from build123d import *

# Parameters (mm, degrees)
SKETCH1_R           = 1.650000007
BOSS_EXTRUDE1_DEPTH = 1
SKETCH9_R           = 1.7
CUT_EXTRUDE3_DEPTH  = 2


with BuildPart() as part:
    # Sketch1 → Boss-Extrude1 (new, symmetric)
    with BuildSketch(Plane(origin=(0, 0, 0), x_dir=(1, 0, 0), z_dir=(0, 1, 0))):
        with BuildLine():
            Line((-3.163944782, -93.076388076), (-20.805834618, -116.891940565))
            ThreePointArc((-20.805834618, -116.891940565), (-21.362478255, -119.119545961), (-20.180929864, -121.088307332))
            Line((-20.180929864, -121.088307332), (-6.520660553, -131.207449705))
            ThreePointArc((-6.520660553, -131.207449705), (-4.293055157, -131.764093342), (-2.324293786, -130.582544951))
            Line((-2.324293786, -130.582544951), (15.317595998, -106.766992534))
            ThreePointArc((15.317595998, -106.766992534), (16.298016652, -105.915587831), (17.546382486, -105.558240139))
            ThreePointArc((17.546382486, -105.558240139), (18.880171652, -105.241928098), (20.028844772, -104.493865997))
            Line((20.028844772, -104.493865997), (31.933718152, -88.422960925))
            ThreePointArc((31.933718152, -88.422960925), (32.812947077, -83.759740105), (28.619624318, -81.538318002))
            Line((28.619624318, -81.538318002), (0.643845867, -85.704349694))
            ThreePointArc((0.643845867, -85.704349694), (-2.081865152, -87.422063847), (-2.657041002, -90.592113564))
            ThreePointArc((-2.657041002, -90.592113564), (-2.635147269, -91.890433717), (-3.163944782, -93.076388076))
        make_face()
        with Locations(Location((1.233011719, -89.660722224, 0), (0, 0, 90))):
            Circle(SKETCH1_R, mode=Mode.SUBTRACT)
        with Locations(Location((29.20879017, -85.494690532, 0), (0, 0, 90))):
            Circle(SKETCH1_R, mode=Mode.SUBTRACT)
        with Locations(Location((17.30391679, -101.565595604, 0), (0, 0, 90))):
            Circle(SKETCH1_R, mode=Mode.SUBTRACT)
    extrude(amount=BOSS_EXTRUDE1_DEPTH, both=True)

    # Sketch9 → Cut-Extrude3 (cut)
    with BuildSketch(Plane(origin=(0, 1, 0), x_dir=(1, 0, 0), z_dir=(0, 1, 0))):
        with Locations(Location((-6.267193351, -106.505511433, 0), (0, 0, 270))):
            Circle(SKETCH9_R)
        with Locations(Location((-14.600604716, -117.755144983, 0), (0, 0, 270))):
            Circle(SKETCH9_R)
        with Locations(Location((-4.958061673, -124.898069011, 0), (0, 0, 270))):
            Circle(SKETCH9_R)
        with Locations(Location((3.375349692, -113.648435461, 0), (0, 0, 270))):
            Circle(SKETCH9_R)
    extrude(amount=-CUT_EXTRUDE3_DEPTH, mode=Mode.SUBTRACT)


solid = part.part
Could you check a few things on this model? Use its own coordinates, in mm. Round coordinates to 2 decimals unless told otherwise and drop trailing zeros. Write each loop counter-clockwise with the first axis right and the second up, starting at its lowest first coordinate (ties: lowest second). Pieces come first, ordered by that corner, then holes. Notation, with made-up numbers: (81.25, 67.25) - (119.25, 67.25) arc R34 cw to (119.25, 99.25) - close; hole circle Ø4 at (73, 68). An arc over 180 degrees is marked (long way). Put each result on its own line as item: value. Start each with the question number.
(1) I want a section at A-A, the plane y = 0.35. Please give me the cut outline in (x, z).
(2) I want a section at C-C, the plane x = 25. Please give me the cut outline in (y, z).
(3) I want a section at D-D, the plane x = 8.5. Please give me the cut outline in (y, z).
(4) Will this pin go through, and if not, where does the flat tip stop? pin 1 (3 mm diameter, centred on x = -14.6, z = 117.76, fed in from +Y).
(5) I want a section at B-B, the plane z = 114. Please give me the cut outline in (x, y).
(6) I need wall thicknesses on probe 1 along X at (y, z) = (0.4, 107.5); probe 2 along X at (y, z) = (0.2, 86); probe 3 along Z at (x, y) = (3.5, -0.4). Which ranges of each line are inside material? Lowest first, please.
(7) Thinking about a two-plate mould opening in X: for faces 1 (the cylindrical face through (-21.367, 0.014, 119.087)), 2 (the cylindrical face through (-4.33, 0.01, 131.77)), 3 (the cylindrical face through (1.865, -0.014, 88.137)), 4 (the cylindrical face through (-6.918, 0.014, 108.076)), which applies, released by +X, released by -X, zero draft, split by the parting line, or undercut?
Here are the results:
1. outline: (-20.81, 116.89) - (-3.16, 93.08) arc R3 cw to (-2.66, 90.59) arc R4 ccw to (0.64, 85.7) - (28.62, 81.54) arc R4 ccw to (31.93, 88.42) - (20.03, 104.49) arc R4 ccw to (17.55, 105.56) arc R3 cw to (15.32, 106.77) - (-2.32, 130.58) arc R3 ccw to (-6.52, 131.21) - (-20.18, 121.09) arc R3 ccw to start; hole circle Ø3.4 at (-14.6, 117.76); hole circle Ø3.4 at (-6.27, 106.51); hole circle Ø3.4 at (-4.96, 124.9); hole circle Ø3.3 at (1.23, 89.66); hole circle Ø3.4 at (3.38, 113.65); hole circle Ø3.3 at (17.3, 101.57); hole circle Ø3.3 at (29.21, 85.49)
2. outline: (-1, 82.08) - (1, 82.08) - (1, 97.78) - (-1, 97.78) - close
3. outline: (-1, 84.53) - (1, 84.53) - (1, 115.97) - (-1, 115.97) - close
4. pin 1: passes through
5. outline: (-18.66, -1) - (1.71, -1) - (1.71, 1) - (-18.66, 1) - close; (5.04, -1) - (9.96, -1) - (9.96, 1) - (5.04, 1) - close
6. probe 1: x = -13.85 to -7.65, -4.89 to 14.77
6. probe 2: x = -0.38 to 27.64, 30.78 to 33.18
6. probe 3: z = 85.28 to 111.95, 115.34 to 122.72
7. face 1: released by -X
7. face 2: split by the parting line
7. face 3: undercut
7. face 4: undercut
